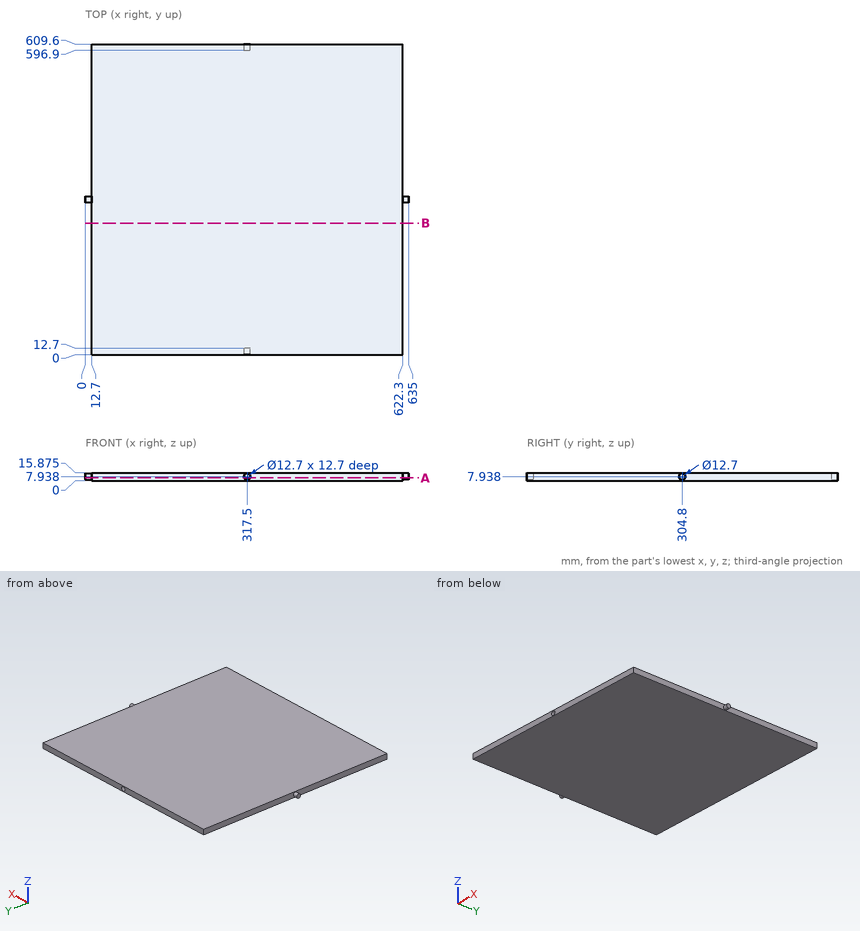
Geometry check sheet. Reference: drawing and pictorial views, mm from the part's lowest x, y, z. Round coordinates to 2 decimals unless told otherwise and drop trailing zeros. Write each loop counter-clockwise with the first axis right and the second up, starting at its lowest first coordinate (ties: lowest second). Pieces come first, ordered by that corner, then holes. Notation, with made-up numbers: (-6.75, -29.75) -> (38.25, -29.75) arc R21 ccw to (38.25, 9.25) -> close; hole circle Ø5 at (45, 28.5). An arc over 180 degrees is marked (long way). One line per question, with ' | ' between items. Start each with the question number.
1. Depth check by flat-ended pin: pin 1 (7.5 mm diameter, centred on x = 317.5, z = 7.94, fed in from -Y); pin 2 (4 mm diameter, centred on x = 317, z = 10.5, fed in from +Y); pin 3 (5 mm diameter, centred on y = 441.5, z = 9.5, fed in from +X). Enter the tip coordinate at first touch or a pass-through.
2. Sectioned sample at B-B, the plane y = 258. Record the cut outline in (x, z) (1 decimal), then the cut area to 3 significant figures.
3. Scan lines: line 1 along Z through (x, y) = (317.5, 4.75) (1 decimal); line 2 along X through (y, z) = (240.5, 9.75); line 3 along Y through (x, z) = (316.5, 7). Record each from-to range of solid material in increasing order. Write a range as from..to.
4. Sectioned sample at A-A, the plane z = 5.25. Record the cut outline in (x, y).
Taken from the geometry:
1) pin 1: stops at y = 12.7 | pin 2: stops at y = 596.9 | pin 3: stops at x = 622.3
2) outline: (12.7, 0) -> (622.3, 0) -> (622.3, 15.9) -> (12.7, 15.9) -> close | area: 9,680 mm^2
3) line 1: z = 0..1.6, 14.3..15.9 | line 2: x = 12.7..622.3 | line 3: y = 12.7..596.9
4) outline: (0, 299.05) -> (12.7, 299.05) -> (12.7, 0) -> (311.75, 0) -> (311.75, 12.7) -> (323.25, 12.7) -> (323.25, 0) -> (622.3, 0) -> (622.3, 299.05) -> (635, 299.05) -> (635, 310.55) -> (622.3, 310.55) -> (622.3, 609.6) -> (323.25, 609.6) -> (323.25, 596.9) -> (311.75, 596.9) -> (311.75, 609.6) -> (12.7, 609.6) -> (12.7, 310.55) -> (0, 310.55) -> close
